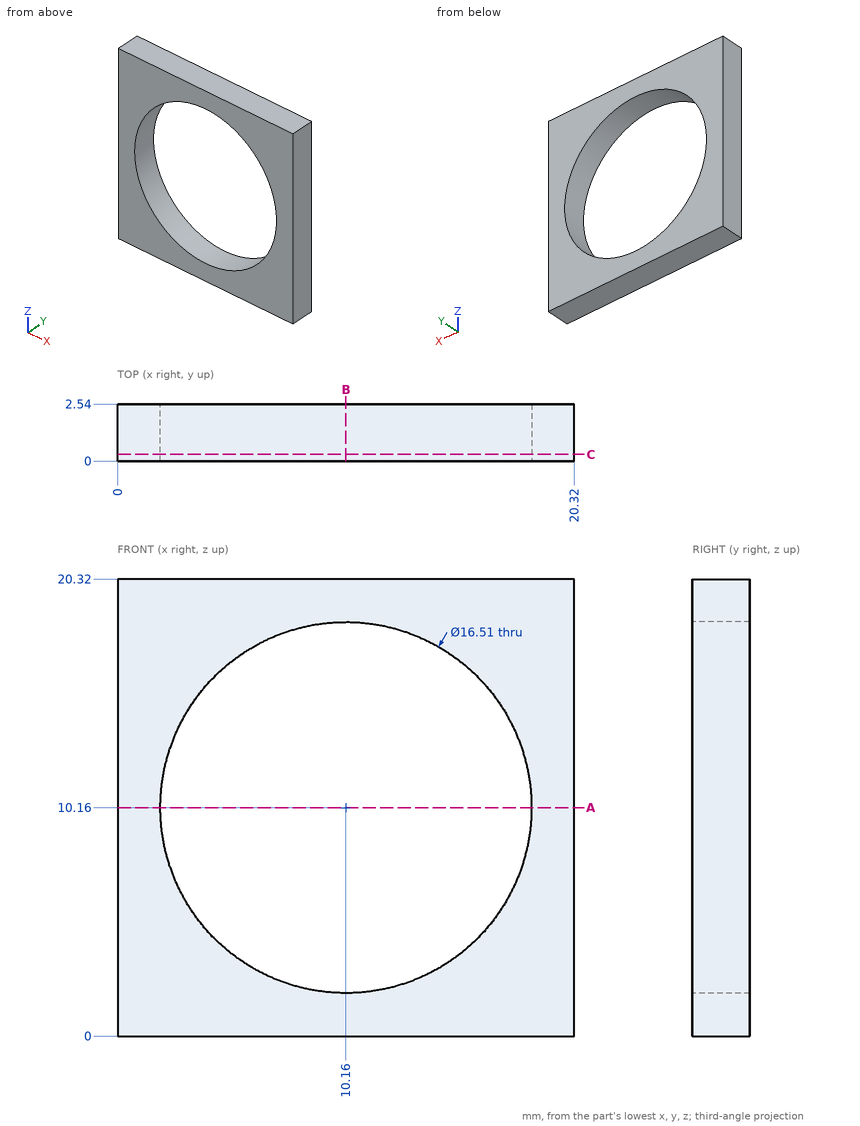
The drawing under review shows one solid part. Ordinate dimensions are in mm from its lowest x, y, z. Give positions to 0.01 mm unless a question says otherwise; leave off trailing zeros. Order: outer loops, then holes, each group sorted by start corner. A loop starts at its lowest first (then second) coordinate and runs counter-clockwise, first axis right, second up. Notation, with made-up numbers: M 64.25,88.25 L 84.25,88.25 A23 cw 84.25,127.25 Z; hole C -33.5,13 d1. An arc over 180 degrees is marked long. Answer in a Markdown table with one row per item. Add a question column.
1. Add section B-B on x = 10.16. State the section outline as (y, z) points (3 decimals).
2. Add section A-A on z = 10.16. State the section outline as (x, y) points (3 decimals).
3. To check wall thickness, follow line 1 along Z through (x, y) = (10.16, 1.65) (3 decimals); line 2 along X through (y, z) = (0.55, 8.75); line 3 along X through (y, z) = (2.35, 5). State the ranges of each line that lie inside material, in increasing order.
4. For pin 1 Ø3 at (x, z) = (14.5, 12.5) entering from -Y, flat-tipped, find the tip position at first contact; note if it passes through.
5. Add section C-C on y = 0.3. State the section outline as (x, z) points (3 decimals).
The answers:
| question | item | result |
|---|---|---|
| 1 | outline | M 0,0 L 2.54,0 L 2.54,1.905 L 0,1.905 Z; M 0,18.415 L 2.54,18.415 L 2.54,20.32 L 0,20.32 Z |
| 2 | outline | M 0,0 L 1.905,0 L 1.905,2.54 L 0,2.54 Z; M 18.415,0 L 20.32,0 L 20.32,2.54 L 18.415,2.54 Z |
| 3 | line 1 | 0 to 1.905, 18.415 to 20.32 |
| 3 | line 2 | 0 to 2.03, 18.29 to 20.32 |
| 3 | line 3 | 0 to 3.72, 16.6 to 20.32 |
| 4 | pin 1 | through |
| 5 | outline | M 0,0 L 20.32,0 L 20.32,20.32 L 0,20.32 Z; hole C 10.16,10.16 d16.51 |
